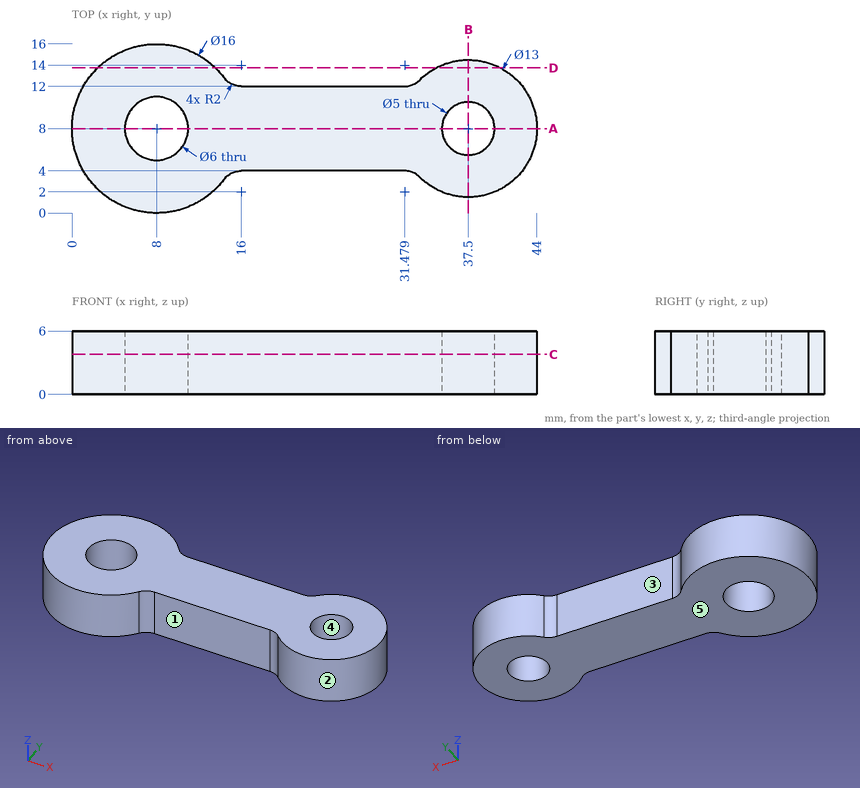
Geometry check sheet. Reference: drawing and pictorial views, mm from the part's lowest x, y, z. A direction names the side the tool comes from. Round coordinates to 2 decimals unless told otherwise and drop trailing zeros. Loops run counter-clockwise (first coordinate to the right, second up) from the corner with the lowest first, then second, coordinate; pieces in that order, holes last. Notation, with made-up numbers: (80, 53.5) - (115, 53.5) arc R16 cw to (115, 60.5) - close; hole circle Ø9 at (-27, 10). An arc over 180 degrees is marked (long way). Answer in a Markdown table with one row per item. Add a question column.
Q1. Release check for a two-part mould opening along X. For the marked faces 4 and 5 record: pulls with the +X half, pulls with the -X half, needs draft (parallel to the pull), parting line crosses it, or undercut.
Q2. Material ranges on line 1 (X direction, y = 8, z = 3.3); line 2 (X direction, y = 5.75, z = 3.4) (1 decimal); line 3 (Y direction, x = 37.5, z = 4.55), recorded low to high.
Q3. Section check B-B on x = 37.5. Enter the section's corners in (y, z), plus the area to 3 significant figures.
Q4. Section check D-D on y = 13.75. Enter the section's corners in (x, z), plus the area to 3 significant figures.
Q5. Tool access check on the marked faces 1, 2 and 3. Record the directions out of +Z, -Z, +X, -X, +Y, -Y that give a thin tool (end or side, any length) a straight path to the whole face; none if there is none.
Q6. Gauge pin test, flat ends, axial feed: pin 1 (1.5 mm diameter, centred on x = 38, z = 5, fed in from -Y); pin 2 (1.5 mm diameter, centred on y = 5.5, z = 3.5, fed in from +X); pin 3 (3 mm diameter, centred on y = 6.5, z = 1.5, fed in from +X); pin 4 (3 mm diameter, centred on x = 24, z = 2, fed in from -Y). Record the tip position at first contact, or that the pin passes through.
Q7. Section check C-C on z = 3.8. Enter the section's corners in (x, y).
Q8. Section check A-A on y = 8. Enter the section's corners in (x, z).
Found:
| question | item | result |
|---|---|---|
| 1 | face 4 | undercut |
| 1 | face 5 | needs draft |
| 2 | line 1 | x = 0 to 5, 11 to 35, 40 to 44 |
| 2 | line 2 | x = 0.3 to 6, 10 to 36.4, 38.6 to 43.6 |
| 2 | line 3 | y = 1.5 to 5.5, 10.5 to 14.5 |
| 3 | outline | (1.5, 0) - (5.5, 0) - (5.5, 6) - (1.5, 6) - close; (10.5, 0) - (14.5, 0) - (14.5, 6) - (10.5, 6) - close |
| 3 | area | 48.0 mm² |
| 4 | outline | (2.44, 0) - (13.56, 0) - (13.56, 6) - (2.44, 6) - close; (34.47, 0) - (40.53, 0) - (40.53, 6) - (34.47, 6) - close |
| 4 | area | 103 mm² |
| 5 | face 1 | +Z, -Z, -Y |
| 5 | face 2 | +Z, -Z |
| 5 | face 3 | +Z, -Z, +Y |
| 6 | pin 1 | stops at y = 1.5 |
| 6 | pin 2 | stops at x = 43.76 |
| 6 | pin 3 | stops at x = 44 |
| 6 | pin 4 | stops at y = 4 |
| 7 | outline | (14.4, 3.2) arc R2 cw to (16, 4) - (31.48, 4) arc R2 cw to (32.9, 3.41) arc R6.5 ccw (long way) to (32.9, 12.59) arc R2 cw to (31.48, 12) - (16, 12) arc R2 cw to (14.4, 12.8) arc R8 ccw (long way) to start; hole circle Ø6 at (8, 8); hole circle Ø5 at (37.5, 8) |
| 8 | outline | (0, 0) - (5, 0) - (5, 6) - (0, 6) - close; (11, 0) - (35, 0) - (35, 6) - (11, 6) - close; (40, 0) - (44, 0) - (44, 6) - (40, 6) - close |
